Source: CAD feature listing. Evaluate the final solid. Frame: model axes, mm. A direction names the side the tool comes from. Round coordinates to 2 decimals unless told otherwise and drop trailing zeros. Loops run counter-clockwise (first coordinate to the right, second up) from the corner with the lowest first, then second, coordinate; pieces in that order, holes last.
(1) Section A-A, the plane y = -12.7. Return the cut outline in (x, z).
(2) Section C-C, the plane x = -1. Return the cut outline in (y, z).
(3) Section B-B, the plane z = 0. Return the cut outline in (x, y).
(4) Mould query, pull axis Z, two halves, no side actions, for faces 1 (the flat face through (6, -13, 37.962)), 2 (the flat face through (6, 0, 17)), 3 (the cylindrical face through (3.45, -12.88, -15.61)). Classes: pulls with the +Z half, pulls with the -Z half, needs draft (parallel to the pull), parting line crosses it, or undercut.
(5) Material intervals for probe 1 along Z at (x, y) = (6.5, -14); probe 2 along Z at (x, y) = (15, -9.25); probe 3 along X at (y, z) = (-4.75, -10), sorted ascending.
(6) Set-up query: faces 4 (the flat face through (6, -25.4, 17)), 5 (the cylindrical face through (-31.646, -9.162, 34.443)). Return all of +Z, -Z, +X, -X, +Y, -Y with unobstructed straight access to the full face (end or side cutting, diameter ignored); none if empty.
(7) Section D-D, the plane x = -33.5. Return the cut outline in (y, z).
```python
from build123d import *

# Parameters (mm, degrees)
F0_W     = 95.25
F0_H     = 76.2
F1_DEPTH = 25.4
F2_R     = 15.99114
F3_DEPTH = 47.498
F4_R     = 3.5687
F5_DEPTH = 7.1374


with BuildPart() as f1:
    # F0 (on Front) → F1 (new body)
    with BuildSketch(Plane.XZ):
        with Locations((6.918825, -0.13822)):
            Rectangle(F0_W, F0_H)
    extrude(amount=F1_DEPTH)

    # F2 (on face) → F3 (cut)
    with BuildSketch(Plane.XZ.offset(25.4)):
        with Locations((6.918825, 0)):
            Circle(F2_R)
    extrude(amount=-F3_DEPTH, mode=Mode.SUBTRACT)

    # F4 (on face) → F5 (cut)
    with BuildSketch(Plane.XY.offset(37.96178)):
        with Locations((-31.181175, -12.7)):
            Circle(F4_R)
        with BuildLine():
            ThreePointArc((41.450125, -12.7), (45.018825, -16.2687), (48.587525, -12.7))
            ThreePointArc((48.587525, -12.7), (45.018825, -9.1313), (41.450125, -12.7))
        make_face()
    extrude(amount=-F5_DEPTH, mode=Mode.SUBTRACT)


solid = f1.part
```
Output values:
1. outline: (-40.71, -38.24) - (54.54, -38.24) - (54.54, 37.96) - (48.59, 37.96) - (48.59, 30.82) - (41.45, 30.82) - (41.45, 37.96) - (-27.61, 37.96) - (-27.61, 30.82) - (-34.75, 30.82) - (-34.75, 37.96) - (-40.71, 37.96) - close; hole circle Ø31.98 at (6.92, 0)
2. outline: (-25.4, -38.24) - (0, -38.24) - (0, -13.89) - (-25.4, -13.89) - close; (-25.4, 13.89) - (0, 13.89) - (0, 37.96) - (-25.4, 37.96) - close
3. outline: (-40.71, -25.4) - (-9.07, -25.4) - (-9.07, 0) - (-40.71, 0) - close; (22.91, -25.4) - (54.54, -25.4) - (54.54, 0) - (22.91, 0) - close
4. face 1: pulls with the +Z half
4. face 2: needs draft
4. face 3: undercut
5. probe 1: z = -38.24 to -15.99, 15.99 to 37.96
5. probe 2: z = -38.24 to -13.8, 13.8 to 37.96
5. probe 3: x = -40.71 to -5.56, 19.4 to 54.54
6. face 4: +Z, -Z, +X, -X, -Y
6. face 5: +Z
7. outline: (-25.4, -38.24) - (0, -38.24) - (0, 37.96) - (-9.99, 37.96) - (-9.99, 30.82) - (-15.41, 30.82) - (-15.41, 37.96) - (-25.4, 37.96) - close
